Study the drawing (mm; zero at the part's minimum x, y, z) and answer. A direction names the side the tool comes from. Coordinates: 2 decimals unless noted, no trailing zeros. Write each loop counter-clockwise with the first axis right and the second up, starting at its lowest first coordinate (ties: lowest second). Pieces come first, ordered by that corner, then holes. Notation, with made-up numbers: (66.25, 52) -> (74.25, 52) arc R18 ccw to (74.25, 72) -> close; hole circle Ø10 at (7.25, -30.5). An arc over 180 degrees is marked (long way). Answer in a Markdown table with one row per item. Add a question column.
Item 1: Section A-A on x = 11.5 is taken. Write down the section's boundary in (y, z), then the cut area to 3 significant figures.
Item 2: Section D-D on x = 20.5 is taken. Write down the section's boundary in (y, z).
Item 3: Straight lines are drawn through the part: line 1 (X direction, y = 3.25, z = 11.5); line 2 (Z direction, x = 11, y = 0.75) (1 decimal); line 3 (Z direction, x = 11.25, y = 2.75) (1 decimal). For each, find the intervals that lie inside material, in ascending order. Write a range as from..to.
Item 4: Section B-B on z = 11.5 is taken. Write down the section's boundary in (x, y), then the cut area to 3 significant figures.
Item 5: Given pin 1 Ø4 at (x, z) = (20.96, 11.5) entering from -Y; pin 2 Ø2 at (y, z) = (3, 16.5) entering from +X; pin 3 Ø2 at (x, y) = (4.5, 5) entering from -Z; pin 4 Ø4.5 at (x, z) = (9.5, 12) entering from -Y, each flat-ended and moving along its own axis, determine where each tip first touches the part or whether it passes through.
Item 6: Which of the six approach directions +Z, -Z, +X, -X, +Y, -Y give full straight-line access (tool end or side, diameter ignored) to the marked faces 4 and 5?
Item 7: For a pull along X with two mould halves and no side action, classify the marked faces 1, 2 and 3 as +X half, -X half, draft (parallel to the pull), parting line (faces both ways), or undercut.
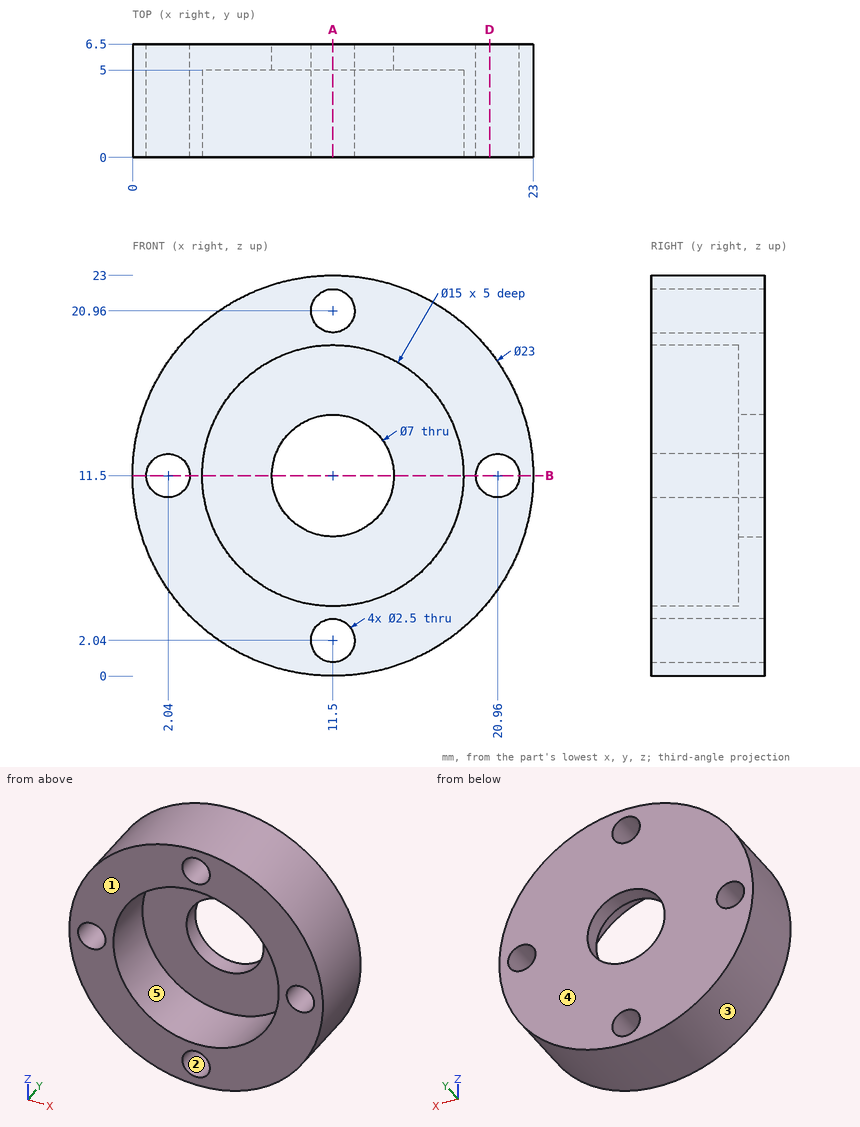
Results below:
| question | item | result |
|---|---|---|
| 1 | outline | (0, 0) -> (6.5, 0) -> (6.5, 0.79) -> (0, 0.79) -> close; (0, 3.29) -> (6.5, 3.29) -> (6.5, 8) -> (5, 8) -> (5, 4) -> (0, 4) -> close; (0, 19) -> (5, 19) -> (5, 15) -> (6.5, 15) -> (6.5, 19.71) -> (0, 19.71) -> close; (0, 22.21) -> (6.5, 22.21) -> (6.5, 23) -> (0, 23) -> close |
| 1 | area | 31.5 mm2 |
| 2 | outline | (0, 4.34) -> (6.5, 4.34) -> (6.5, 10.34) -> (0, 10.34) -> close; (0, 12.66) -> (6.5, 12.66) -> (6.5, 18.66) -> (0, 18.66) -> close |
| 3 | line 1 | x = 0..0.79, 3.29..4, 19..19.71, 22.21..23 |
| 3 | line 2 | z = 0..0.9, 3.2..4, 19..19.8, 22.1..23 |
| 3 | line 3 | z = 0..0.8, 3.3..4, 19..19.7, 22.2..23 |
| 4 | outline | (0, 0) -> (0.79, 0) -> (0.79, 6.5) -> (0, 6.5) -> close; (3.29, 0) -> (4, 0) -> (4, 5) -> (8, 5) -> (8, 6.5) -> (3.29, 6.5) -> close; (15, 5) -> (19, 5) -> (19, 0) -> (19.71, 0) -> (19.71, 6.5) -> (15, 6.5) -> close; (22.21, 0) -> (23, 0) -> (23, 6.5) -> (22.21, 6.5) -> close |
| 4 | area | 31.5 mm2 |
| 5 | pin 1 | stops at y = 0 |
| 5 | pin 2 | stops at x = 22.28 |
| 5 | pin 3 | stops at z = 1.69 |
| 5 | pin 4 | stops at y = 5 |
| 6 | face 4 | +Z, -Z, +X, -X, +Y |
| 6 | face 5 | -Y |
| 7 | face 1 | draft |
| 7 | face 2 | undercut |
| 7 | face 3 | parting line |
